```python
from build123d import *

# Parameters (mm, degrees)
BOSS_EXTRUDE1_OUTLINE_R   = 1
BOSS_EXTRUDE1_OUTLINE_W   = 5
BOSS_EXTRUDE1_OUTLINE_H   = 5
BOSS_EXTRUDE1_OUTLINE_R_2 = 1.5
BOSS_EXTRUDE1_OUTLINE_R_3 = 4.05
BOSS_EXTRUDE1_DEPTH       = 2
CONG_1_R                  = 5


# Read off the part's stored shape, not the designer's step: Boss-Extrude1
with BuildPart() as part:
    # Boss-Extrude1 outline → Boss-Extrude1 (new body)
    with BuildSketch(Plane.XY):
        with BuildLine():
            Line((46, -11.7), (46, 11.7))
            Line((46, 11.7), (0, 11.7))
            ThreePointArc((0, 11.7), (-11.7, 0), (0, -11.7))
            Line((0, -11.7), (46, -11.7))
        make_face()
        with Locations((-3.5, -6.062177826)):
            Circle(BOSS_EXTRUDE1_OUTLINE_R, mode=Mode.SUBTRACT)
        with Locations((0, -7)):
            Circle(BOSS_EXTRUDE1_OUTLINE_R, mode=Mode.SUBTRACT)
        with Locations((3.5, -6.062177826)):
            Circle(BOSS_EXTRUDE1_OUTLINE_R, mode=Mode.SUBTRACT)
        with Locations((-6.062177826, -3.5)):
            Circle(BOSS_EXTRUDE1_OUTLINE_R, mode=Mode.SUBTRACT)
        with Locations((6.062177826, -3.5)):
            Circle(BOSS_EXTRUDE1_OUTLINE_R, mode=Mode.SUBTRACT)
        with Locations((25.5, -5)):
            Rectangle(BOSS_EXTRUDE1_OUTLINE_W, BOSS_EXTRUDE1_OUTLINE_H, mode=Mode.SUBTRACT)
        with Locations((33, -5)):
            Circle(BOSS_EXTRUDE1_OUTLINE_R_2, mode=Mode.SUBTRACT)
        with Locations((40.5, -5)):
            Rectangle(BOSS_EXTRUDE1_OUTLINE_W, BOSS_EXTRUDE1_OUTLINE_H, mode=Mode.SUBTRACT)
        with Locations((-7, 0)):
            Circle(BOSS_EXTRUDE1_OUTLINE_R, mode=Mode.SUBTRACT)
        Circle(BOSS_EXTRUDE1_OUTLINE_R_3, mode=Mode.SUBTRACT)
        with Locations((-6.062177826, 3.5)):
            Circle(BOSS_EXTRUDE1_OUTLINE_R, mode=Mode.SUBTRACT)
        with Locations((7, 0)):
            Circle(BOSS_EXTRUDE1_OUTLINE_R, mode=Mode.SUBTRACT)
        with Locations((6.062177826, 3.5)):
            Circle(BOSS_EXTRUDE1_OUTLINE_R, mode=Mode.SUBTRACT)
        with Locations((-3.5, 6.062177826)):
            Circle(BOSS_EXTRUDE1_OUTLINE_R, mode=Mode.SUBTRACT)
        with Locations((0, 7)):
            Circle(BOSS_EXTRUDE1_OUTLINE_R, mode=Mode.SUBTRACT)
        with Locations((3.5, 6.062177826)):
            Circle(BOSS_EXTRUDE1_OUTLINE_R, mode=Mode.SUBTRACT)
        with Locations((25.5, 5)):
            Rectangle(BOSS_EXTRUDE1_OUTLINE_W, BOSS_EXTRUDE1_OUTLINE_H, mode=Mode.SUBTRACT)
        with Locations((33, 5)):
            Circle(BOSS_EXTRUDE1_OUTLINE_R_2, mode=Mode.SUBTRACT)
        with Locations((40.5, 5)):
            Rectangle(BOSS_EXTRUDE1_OUTLINE_W, BOSS_EXTRUDE1_OUTLINE_H, mode=Mode.SUBTRACT)
    extrude(amount=BOSS_EXTRUDE1_DEPTH)

    # Congé1
    cong_1_edges = [part.edges().sort_by_distance(p)[0] for p in [
        (46, 11.7, 1),
        (46, -11.7, 1),
    ]]
    fillet(cong_1_edges, radius=CONG_1_R)


solid = part.part
```
Here's how the part is built. I have some questions about the finished solid (model axes, mm). A direction names the side the tool comes from. Give positions to 0.01 mm unless a question says otherwise; leave off trailing zeros. Order: outer loops, then holes, each group sorted by start corner. A loop starts at its lowest first (then second) coordinate and runs counter-clockwise, first axis right, second up. Notation, with made-up numbers: M -1,59.25 L 9,59.25 A25 ccw 9,87.25 Z; hole C 41.5,-13 d3. An arc over 180 degrees is marked long. Use a Markdown table: item, result. Add a question column.
1. For pin 1 Ø1.6 at (x, y) = (-7, 0) entering from -Z; pin 2 Ø1 at (y, z) = (6.5, 1) entering from -X; pin 3 Ø1 at (y, z) = (4, 1.5) entering from -X, each with a flat end and sliding along its axis, tell me the tip position at first contact or that it passes through.
2. If we mould it in two halves opening along X, with no side actions, what happens to faces 3 (the flat face through (17, 0, 0)), 4 (the flat face through (46, 0, 1)), 5 (the cylindrical face through (6.2, -0.6, 1))? For each: +X half, -X half, draft (parallel to the pull), parting line (faces both ways), or undercut.
3. Suppose I cut it at B-B (y = 1.75). List the corners of the cut face in (x, z) for me.
4. Suppose I cut it at A-A (x = 33). List the corners of the cut face in (y, z) for me.
5. I need wall thicknesses on probe 1 along Y at (x, z) = (0, 0.9); probe 2 along Y at (x, z) = (39, 1.7); probe 3 along Y at (x, z) = (32.5, 0.6). Which ranges of each line are inside material? Lowest first, please. Write a range as from..to.
6. On a 3-axis mill with a long thin cutter (end or side, diameter ignored), from which of +Z, -Z, +X, -X, +Y, -Y can I reach the whole of each face in a straight line? I mean faces 1 (the flat face through (17, 0, 2)), 2 (the flat face through (40, -2.5, 1)). Say none if no direction works.
7. Suppose I cut it at C-C (x = 3.5). List the corners of the cut face in (y, z) for me, and give its area (3 significant figures).
8. Suppose I cut it at D-D (z = 1.3). Give the number of separate pieces and of enclosed holes in the cut face, and give its area (3 significant figures).
Results list:
| question | item | result |
|---|---|---|
| 1 | pin 1 | passes through |
| 1 | pin 2 | stops at x = -10.04 |
| 1 | pin 3 | stops at x = -11.16 |
| 2 | face 3 | draft |
| 2 | face 4 | +X half |
| 2 | face 5 | undercut |
| 3 | outline | M -11.57,0 L -3.65,0 L -3.65,2 L -11.57,2 Z; M 3.65,0 L 46,0 L 46,2 L 3.65,2 Z |
| 4 | outline | M -11.7,0 L -6.5,0 L -6.5,2 L -11.7,2 Z; M -3.5,0 L 3.5,0 L 3.5,2 L -3.5,2 Z; M 6.5,0 L 11.7,0 L 11.7,2 L 6.5,2 Z |
| 5 | probe 1 | y = -11.7..-8, -6..-4.05, 4.05..6, 8..11.7 |
| 5 | probe 2 | y = -11.7..-7.5, -2.5..2.5, 7.5..11.7 |
| 5 | probe 3 | y = -11.7..-6.41, -3.59..3.59, 6.41..11.7 |
| 6 | face 1 | +Z, +X, -X, +Y, -Y |
| 6 | face 2 | +Z, -Z |
| 7 | outline | M -11.7,0 L -7.06,0 L -7.06,2 L -11.7,2 Z; M -5.06,0 L -2.04,0 L -2.04,2 L -5.06,2 Z; M 2.04,0 L 5.06,0 L 5.06,2 L 2.04,2 Z; M 7.06,0 L 11.7,0 L 11.7,2 L 7.06,2 Z |
| 7 | area | 30.6 mm² |
| 8 | separate pieces | 1 |
| 8 | enclosed holes | 19 |
| 8 | area | 1,080 mm² |
